from build123d import *

# Parameters (mm, degrees)
SKETCH1_W           = 102.3
SKETCH1_H           = 52
BOSS_EXTRUDE1_DEPTH = 5
CUT_EXTRUDE1_DEPTH  = 5
CUT_EXTRUDE2_DEPTH  = 10
SKETCH9_R           = 4.2
CUT_EXTRUDE3_DEPTH  = 5


with BuildPart() as part:
    # Sketch1 → Boss-Extrude1 (new body)
    with BuildSketch(Plane.XY):
        Rectangle(SKETCH1_W, SKETCH1_H)
    extrude(amount=BOSS_EXTRUDE1_DEPTH)

    # Sketch3 → Cut-Extrude1 (cut)
    with BuildSketch(Plane.XY.offset(5)):
        Polygon((-36.65, 17.8), (-36.65, 7.8), (-40.65, 7.8), (-40.65, 17.8), (-42.15, 17.8), (-42.15, 21), (-40.65, 21), (-40.65, 26), (-36.65, 26), (-36.65, 21), (-35.15, 21), (-35.15, 17.8), align=None)
        Polygon((-40.65, -7.8), (-40.65, -17.8), (-42.15, -17.8), (-42.15, -21), (-40.65, -21), (-40.65, -26), (-36.65, -26), (-36.65, -21), (-35.15, -21), (-35.15, -17.8), (-36.65, -17.8), (-36.65, -7.8), align=None)
    extrude(amount=-CUT_EXTRUDE1_DEPTH, mode=Mode.SUBTRACT)

    # Sketch8 → Cut-Extrude2 (cut)
    with BuildSketch(Plane.XY.offset(5)):
        Polygon((36.95, 26), (36.95, 21), (35.45, 21), (35.45, 17.8), (36.95, 17.8), (36.95, 7.8), (40.95, 7.8), (40.95, 17.8), (42.45, 17.8), (42.45, 21), (40.95, 21), (40.95, 26), align=None)
        Polygon((40.95, -17.8), (42.45, -17.8), (42.45, -21), (40.95, -21), (40.95, -26), (36.95, -26), (36.95, -21), (35.45, -21), (35.45, -17.8), (36.95, -17.8), (36.95, -7.8), (40.95, -7.8), align=None)
    extrude(amount=-CUT_EXTRUDE2_DEPTH, mode=Mode.SUBTRACT)

    # Sketch9 → Cut-Extrude3 (cut)
    with BuildSketch(Plane.XY.offset(5)):
        with Locations((0.15, 28.5)):
            Circle(SKETCH9_R)
    extrude(amount=-CUT_EXTRUDE3_DEPTH, mode=Mode.SUBTRACT)


solid = part.part
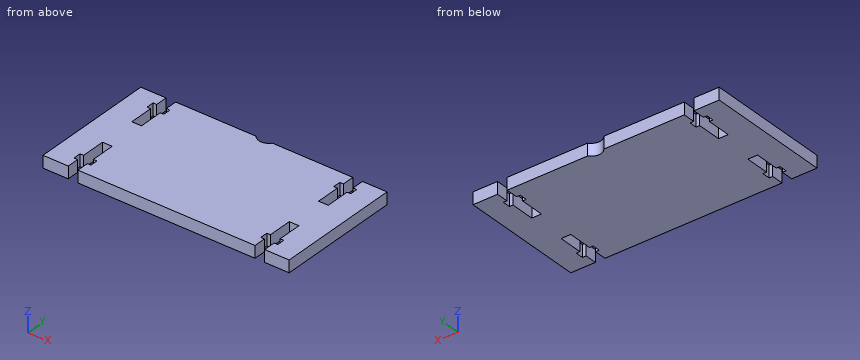
Can you work these out from the model? Positions are in its coordinate system, mm. Coordinates: 2 decimals unless noted, no trailing zeros. Write each loop counter-clockwise with the first axis right and the second up, starting at its lowest first coordinate (ties: lowest second). Pieces come first, ordered by that corner, then holes. Notation, with made-up numbers: (-35, -31.5) -> (-30, -31.5) arc R24 ccw to (-30, -11.5) -> close; hole circle Ø2 at (9.25, -21). An arc over 180 degrees is marked (long way). Write each question's results on one line, items separated by ' | '. Start each with the question number.
Q1. I'm going to push a flat-ended pin straight in: pin 1 (3 mm diameter, centred on x = 39.5, z = 1.5, fed in from -Y). Where does the tip first touch, or does it pass through?
Q2. If I drill on probe 1 along X at (y, z) = (-13, 3.9); probe 2 along X at (y, z) = (-20.5, 3.2); probe 3 along Y at (x, z) = (-39.5, 0.4), over which ranges is the centre line in solid material (lowest first)?
Q3. Imagine slicing it at A-A (y = 20). Write out the boundary of the cut face in (x, z).
Taken from the geometry:
1) pin 1: stops at y = -26
2) probe 1: x = -51.15 to -40.65, -36.65 to 36.95, 40.95 to 51.15 | probe 2: x = -51.15 to -42.15, -35.15 to 35.45, 42.45 to 51.15 | probe 3: y = -7.8 to 7.8
3) outline: (-51.15, 0) -> (-42.15, 0) -> (-42.15, 5) -> (-51.15, 5) -> close; (-35.15, 0) -> (35.45, 0) -> (35.45, 5) -> (-35.15, 5) -> close; (42.45, 0) -> (51.15, 0) -> (51.15, 5) -> (42.45, 5) -> close
